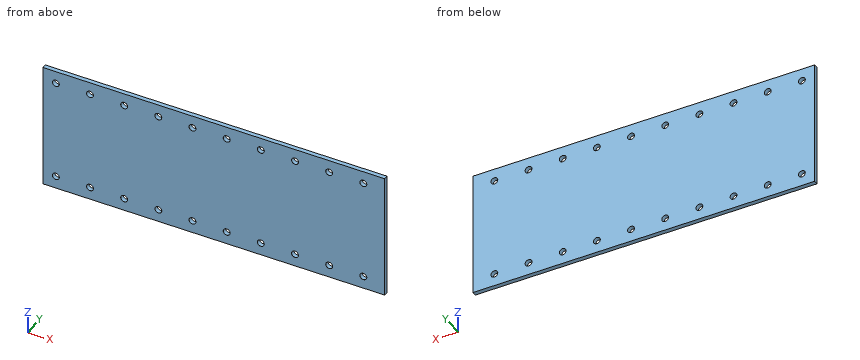
```python
from build123d import *

# Parameters (mm, degrees)
SKETCH1_W                      = 200
SKETCH1_H                      = 75
BOSS_EXTRUDE1_DEPTH            = 2.5
F_4_0MM_DOWEL_HOLE1_AT_2_COUNT = 2
F_4_0MM_DOWEL_HOLE1_AT_2_PITCH = 60
LPATTERN1_COUNT                = 10
LPATTERN1_PITCH                = 20


with BuildPart() as part:
    # Sketch1 → Boss-Extrude1 (new body)
    with BuildSketch(Plane(origin=(0, 0, 0), x_dir=(1, 0, 0), z_dir=(0, 1, 0))):
        Rectangle(SKETCH1_W, SKETCH1_H)
    extrude(amount=BOSS_EXTRUDE1_DEPTH)

    # Sketch4 → Ø4.0mm Dowel Hole1 (revolve, cut)
    with BuildSketch(Plane(origin=(-92.5, 2.5, -30), x_dir=(0, 0, 1), z_dir=(1, 0, 0))):
        Polygon((0, 0), (0, 2.5), (2.025, 2.5), (2, 2.475), (2, 0), align=None)
    f_4_0mm_dowel_hole1 = revolve(axis=Axis((-92.5, 8.85, -30), (0, -1, 0)), mode=Mode.SUBTRACT)

    # Ø4.0mm Dowel Hole1 at 2: Ø4.0mm Dowel Hole1 ×2
    with Locations(*[(0, 0, i * F_4_0MM_DOWEL_HOLE1_AT_2_PITCH) for i in range(1, F_4_0MM_DOWEL_HOLE1_AT_2_COUNT)]):
        add(f_4_0mm_dowel_hole1, mode=Mode.SUBTRACT)

    # LPattern1: Ø4.0mm Dowel Hole1 ×10
    with Locations(*[(i * LPATTERN1_PITCH, 0, 0) for i in range(1, LPATTERN1_COUNT)]):
        add(f_4_0mm_dowel_hole1, mode=Mode.SUBTRACT)

    # LPattern1 copy 1 sketch → LPattern1 copy 1 (revolve, cut)
    with BuildSketch(Plane(origin=(-72.5, 2.5, 30), x_dir=(0, 0, 1), z_dir=(1, 0, 0))):
        Polygon((0, 0), (0, 2.5), (2.025, 2.5), (2, 2.475), (2, 0), align=None)
    revolve(axis=Axis((-72.5, 8.85, 30), (0, -1, 0)), mode=Mode.SUBTRACT)

    # LPattern1 copy 2 sketch → LPattern1 copy 2 (revolve, cut)
    with BuildSketch(Plane(origin=(-52.5, 2.5, 30), x_dir=(0, 0, 1), z_dir=(1, 0, 0))):
        Polygon((0, 0), (0, 2.5), (2.025, 2.5), (2, 2.475), (2, 0), align=None)
    revolve(axis=Axis((-52.5, 8.85, 30), (0, -1, 0)), mode=Mode.SUBTRACT)

    # LPattern1 copy 3 sketch → LPattern1 copy 3 (revolve, cut)
    with BuildSketch(Plane(origin=(-32.5, 2.5, 30), x_dir=(0, 0, 1), z_dir=(1, 0, 0))):
        Polygon((0, 0), (0, 2.5), (2.025, 2.5), (2, 2.475), (2, 0), align=None)
    revolve(axis=Axis((-32.5, 8.85, 30), (0, -1, 0)), mode=Mode.SUBTRACT)

    # LPattern1 copy 4 sketch → LPattern1 copy 4 (revolve, cut)
    with BuildSketch(Plane(origin=(-12.5, 2.5, 30), x_dir=(0, 0, 1), z_dir=(1, 0, 0))):
        Polygon((0, 0), (0, 2.5), (2.025, 2.5), (2, 2.475), (2, 0), align=None)
    revolve(axis=Axis((-12.5, 8.85, 30), (0, -1, 0)), mode=Mode.SUBTRACT)

    # LPattern1 copy 5 sketch → LPattern1 copy 5 (revolve, cut)
    with BuildSketch(Plane(origin=(7.5, 2.5, 30), x_dir=(0, 0, 1), z_dir=(1, 0, 0))):
        Polygon((0, 0), (0, 2.5), (2.025, 2.5), (2, 2.475), (2, 0), align=None)
    revolve(axis=Axis((7.5, 8.85, 30), (0, -1, 0)), mode=Mode.SUBTRACT)

    # LPattern1 copy 6 sketch → LPattern1 copy 6 (revolve, cut)
    with BuildSketch(Plane(origin=(27.5, 2.5, 30), x_dir=(0, 0, 1), z_dir=(1, 0, 0))):
        Polygon((0, 0), (0, 2.5), (2.025, 2.5), (2, 2.475), (2, 0), align=None)
    revolve(axis=Axis((27.5, 8.85, 30), (0, -1, 0)), mode=Mode.SUBTRACT)

    # LPattern1 copy 7 sketch → LPattern1 copy 7 (revolve, cut)
    with BuildSketch(Plane(origin=(47.5, 2.5, 30), x_dir=(0, 0, 1), z_dir=(1, 0, 0))):
        Polygon((0, 0), (0, 2.5), (2.025, 2.5), (2, 2.475), (2, 0), align=None)
    revolve(axis=Axis((47.5, 8.85, 30), (0, -1, 0)), mode=Mode.SUBTRACT)

    # LPattern1 copy 8 sketch → LPattern1 copy 8 (revolve, cut)
    with BuildSketch(Plane(origin=(67.5, 2.5, 30), x_dir=(0, 0, 1), z_dir=(1, 0, 0))):
        Polygon((0, 0), (0, 2.5), (2.025, 2.5), (2, 2.475), (2, 0), align=None)
    revolve(axis=Axis((67.5, 8.85, 30), (0, -1, 0)), mode=Mode.SUBTRACT)

    # LPattern1 copy 9 sketch → LPattern1 copy 9 (revolve, cut)
    with BuildSketch(Plane(origin=(87.5, 2.5, 30), x_dir=(0, 0, 1), z_dir=(1, 0, 0))):
        Polygon((0, 0), (0, 2.5), (2.025, 2.5), (2, 2.475), (2, 0), align=None)
    revolve(axis=Axis((87.5, 8.85, 30), (0, -1, 0)), mode=Mode.SUBTRACT)


solid = part.part
```
Geometry check sheet. Reference: the model listing, model coordinates, mm. Coordinates: 2 decimals unless noted, no trailing zeros. Order: outer loops, then holes, each group sorted by start corner. A loop starts at its lowest first (then second) coordinate and runs counter-clockwise, first axis right, second up. Notation, with made-up numbers: (73.5, -37.75) - (93.5, -37.75) arc R31 cw to (93.5, -2.75) - close; hole circle Ø11 at (15, -18.75). An arc over 180 degrees is marked (long way). Answer as a JSON object with one key per item and string values. Group by question number.
Item 1: Sectioned sample at A-A, the plane x = -12.5. Record the cut outline in (y, z) (3 decimals), and give its area (3 significant figures).
Item 2: Scan lines: probe 1 along Z at (x, y) = (7.5, 1.65); probe 2 along Z at (x, y) = (68, 1.4). Record each from-to range of solid material in increasing order.
Item 3: Sectioned sample at B-B, the plane y = 1.9. Give the number of separate pieces and of enclosed holes in the cut face, and give its area (3 significant figures).
Resolved:
{
 "1": {"outline": "(0, -37.5) - (2.5, -37.5) - (2.5, -32) - (0.025, -32) - (0, -32.025) - close; (0, -27.975) - (0.025, -28) - (2.5, -28) - (2.5, 28) - (0.025, 28) - (0, 27.975) - close; (0, 32.025) - (0.025, 32) - (2.5, 32) - (2.5, 37.5) - (0, 37.5) - close", "area": "167 mm^2"},
 "2": {"probe 1": "-37.5 to -32, -28 to 28, 32 to 37.5", "probe 2": "-37.5 to -31.94, -28.06 to 28.06, 31.94 to 37.5"},
 "3": {"separate pieces": "1", "enclosed holes": "20", "area": "14,700 mm^2"}
}
